Input: part model. Units: mm. Frame: model coordinates. Round coordinates to 2 decimals unless told otherwise and drop trailing zeros. Order: outer loops, then holes, each group sorted by start corner. A loop starts at its lowest first (then second) coordinate and runs counter-clockwise, first axis right, second up. Notation, with made-up numbers: M 13,77.25 L 52,77.25 A19 ccw 52,100.25 Z; hole C 84.25,75 d5. An arc over 180 degrees is marked long. One line per question, with ' | ' between items.
```python
from build123d import *

# Parameters (mm, degrees)
SKETCH1_R           = 76.2
BOSS_EXTRUDE1_DEPTH = 2.54
SKETCH2_R           = 3.175
CUT_EXTRUDE2_DEPTH  = 108.793003484
CIRPATTERN2_COUNT   = 4


with BuildPart() as part:
    # Sketch1 → Boss-Extrude1 (new body)
    with BuildSketch(Plane.YZ):
        with Locations(Location((0, 0, 0), (0, 0, 270))):
            Circle(SKETCH1_R)
    extrude(amount=BOSS_EXTRUDE1_DEPTH)

    # Sketch2 → Cut-Extrude2 (cut, through all)
    with BuildSketch(Plane(origin=(2.54, 0, 0), x_dir=(0, 0, -1), z_dir=(1, 0, 0))):
        with Locations((-62.23, 0)):
            Circle(SKETCH2_R)
    cut_extrude2 = extrude(amount=-CUT_EXTRUDE2_DEPTH, mode=Mode.SUBTRACT)

    # CirPattern2: Cut-Extrude2 ×4 about axis
    cirpattern2_axis = Axis((0, 0, 0), (1, 0, 0))
    for i in range(1, CIRPATTERN2_COUNT):
        add(cut_extrude2.rotate(cirpattern2_axis, i * 360 / CIRPATTERN2_COUNT), mode=Mode.SUBTRACT)


solid = part.part
```
Item 1: Line query: line 1 along Z through (x, y) = (1.65, -62.23) (3 decimals); line 2 along Y through (x, z) = (0.4, 63). Output: solid intervals per line, ascending. Write a range as from..to.
Report:
line 1: -43.976..-3.175, 3.175..43.976 | line 2: -42.87..-3.08, 3.08..42.87
Item 2: Section query C-C, the plane z = -62.23. Return loops of the section in (x, y) (3 decimals), plus the area to 3 significant figures.
Report:
outline: M 0,-43.976 L 2.54,-43.976 L 2.54,-3.175 L 0,-3.175 Z; M 0,3.175 L 2.54,3.175 L 2.54,43.976 L 0,43.976 Z | area: 207 mm²
Item 3: Section query B-B, the plane x = 1.1. Return loops of the section in (y, z) (3 decimals).
Report:
outline: C 0,0 d152.4; hole C -62.23,0 d6.35; hole C 0,-62.23 d6.35; hole C 0,62.23 d6.35; hole C 62.23,0 d6.35
Item 4: Section query A-A, the plane z = 0. Return loops of the section in (x, y) (3 decimals), plus the area to 3 significant figures.
Report:
outline: M 0,-76.2 L 2.54,-76.2 L 2.54,-65.405 L 0,-65.405 Z; M 0,-59.055 L 2.54,-59.055 L 2.54,59.055 L 0,59.055 Z; M 0,65.405 L 2.54,65.405 L 2.54,76.2 L 0,76.2 Z | area: 355 mm²
Item 5: First-contact query: pin 1 (10 mm diameter, centred on y = 0, z = -62.23, fed in from +X); pin 2 (1 mm diameter, centred on x = 1, y = -47, fed in from -Z). Flat tips, straight axial feed; report the tip coordinate or a pass-through.
Report:
pin 1: x = 2.54 | pin 2: z = -60.37
Item 6: Mould query, pull axis Y, two halves, no side actions, for faces 1 (the flat face through (2.54, 1, 1)), 2 (the cylindrical face through (1.29, -59.2, 0.95)), 3 (the cylindrical face through (1.252, -46.367, 60.47)), 4 (the cylindrical face through (1.29, 0.95, 59.2)). Classes: +Y half, -Y half, draft (parallel to the pull), parting line (faces both ways), or undercut.
Report:
face 1: draft | face 2: undercut | face 3: parting line | face 4: undercut
